Verification items for the finished model (mm, model axes). Face numbers are marked on the shaded views. Round coordinates to 2 decimals unless told otherwise and drop trailing zeros. Write each loop counter-clockwise with the first axis right and the second up, starting at its lowest first coordinate (ties: lowest second). Pieces come first, ordered by that corner, then holes. Notation, with made-up numbers: M 38.25,63.5 L 78.25,63.5 A16 cw 78.25,75.5 Z; hole C 15.5,41.5 d9. An arc over 180 degrees is marked long. One line per question, with ' | ' between items. Start each with the question number.
Q1. Release check for a two-part mould opening along X. For the marked faces 1, 2 and 3 record: released by +X, released by -X, zero draft, split by the parting line, or undercut.
Q2. Cross-section at A-A (y = 0). Record the boundary of the cut face in (x, z).
Q3. Gauge pin test, flat ends, axial feed: pin 1 (2 mm diameter, centred on y = 30.5, z = 18, fed in from -X); pin 2 (4 mm diameter, centred on x = 12.5, y = -2.5, fed in from +Z); pin 3 (6 mm diameter, centred on x = 18, z = 8, fed in from +Y). Record the tip position at first contact, or that the pin passes through.
Q4. Cross-section at C-C (z = 38). Record the boundary of the cut face in (x, y).
Q5. Thickness scan on line 1 along Y through (x, z) = (0, 18.5); line 2 along Y through (x, z) = (27, 7.5); line 3 along Z through (x, y) = (-20.5, -5.5). Record the ranges inside material, lowest first. Write a range as from..to.
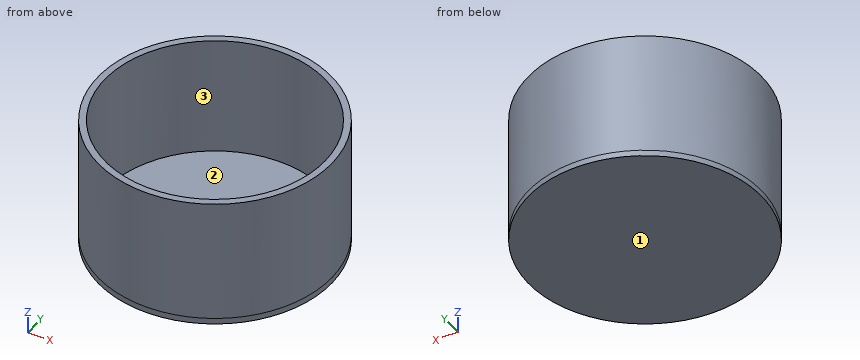
from build123d import *

# Parameters (mm, degrees)
F0_R     = 39
F1_DEPTH = 1.5
F2_R     = 39
F2_R_2   = 36.75
F3_DEPTH = 40
F4_DEPTH = 2


with BuildPart() as f1:
    # F0 (on Top) → F1 (new body)
    with BuildSketch(Plane.XY):
        Circle(F0_R)
    extrude(amount=F1_DEPTH)

    # F2 (on face) → F3 (join)
    with BuildSketch(Plane.XY.offset(1.5)):
        Circle(F2_R)
        Circle(F2_R_2, mode=Mode.SUBTRACT)
    extrude(amount=F3_DEPTH)

    # F4 (add): a face of the model
    f4_faces = [f1.faces().sort_by_distance(p)[0] for p in [
        (0, 0, 0),
    ]]
    extrude(f4_faces, amount=F4_DEPTH)


solid = f1.part
Determined:
1) face 1: zero draft | face 2: undercut | face 3: undercut
2) outline: M -39,-2 L 39,-2 L 39,41.5 L 36.75,41.5 L 36.75,1.5 L -36.75,1.5 L -36.75,41.5 L -39,41.5 Z
3) pin 1: stops at x = -25.51 | pin 2: stops at z = 1.5 | pin 3: stops at y = 36
4) outline: C 0,0 d78; hole C 0,0 d73.5
5) line 1: y = -39..-36.75, 36.75..39 | line 2: y = -28.14..-24.93, 24.93..28.14 | line 3: z = -2..1.5
